Geometry: final body of the model. Coordinates: model frame, mm. Round coordinates to 2 decimals unless told otherwise and drop trailing zeros. Write each loop counter-clockwise with the first axis right and the second up, starting at its lowest first coordinate (ties: lowest second). Pieces come first, ordered by that corner, then holes. Notation, with made-up numbers: M -36.5,47 L 2.5,47 A20 ccw 2.5,75 Z; hole C -18.5,-34.5 d9. An arc over 180 degrees is marked long. Use one line per item in the form item = value. Start each with the question number.
Autodesk Inventor part; units mm, degrees
ref_plane "YZ Plane" through (0, 0, 0) normal (1, 0, 0) x (0, 1, 0)
ref_plane "XZ Plane" through (0, 0, 0) normal (0, 1, 0) x (-1, 0, 0)
ref_plane "XY Plane" through (0, 0, 0) normal (0, 0, 1) x (1, 0, 0)
sketch "Sketch1" plane through (0, 0, 0) normal (0, 0, 1) x (1, 0, 0)
  line L0 (0, 22.2362) -> (22.2362, 22.2362) construction
  line L1 (22.2362, 22.2362) -> (22.2362, 0) construction
  line L2 (22.2362, 0) -> (0, 0)
  line L3 (0, 0) -> (0, 22.2362)
  line L4 (0, 22.2362) -> (22.2362, 0) construction
  line L5 (22.2362, 22.2362) -> (0, 0) construction
  line L6 (208.1103, 421.1181) -> (230.3465, 421.1181)
  line L7 (230.3465, 421.1181) -> (230.3465, 398.8819)
  line L8 (230.3465, 398.8819) -> (208.1103, 398.8819) construction
  line L9 (208.1103, 398.8819) -> (208.1103, 421.1181) construction
  line L10 (208.1103, 421.1181) -> (230.3465, 398.8819) construction
  line L11 (230.3465, 421.1181) -> (208.1103, 398.8819) construction
  line L12 (208.1103, 421.1181) -> (0, 22.2362)
  line L13 (230.3465, 398.8819) -> (22.2362, 0)
  line L14 (0, 0) -> (230.3465, 421.1181) construction
  line L15 (-46.0693, 0) -> (276.4159, 0) construction
  point P0 (11.1181, 11.1181)
  point P1 (219.2284, 410)
  point P2 (115.1733, 210.5591)
  dimension "d1" = 480
  dimension "d14" = 410
  dimension "d15" = 30
extrude "Extrusion1" add sketch "Sketch1" along normal mid plane 10
sketch "Sketch2" plane through (0, 0, 5) normal (0, 0, 1) x (1, 0, 0)
  line L0 (230.3465, 421.1181) -> (208.1103, 421.1181) construction
  line L1 (230.3465, 398.8819) -> (230.3465, 421.1181) construction
  line L2 (208.1103, 421.1181) -> (230.3465, 398.8819) construction
  point P0 (0, 0)
  point P1 (219.2284, 410)
hole "Hole1" at (219.2284, 410, 5) direction (0, 0, -1) diameter 8 end through all
properties part number "Support - Left"
1. Section query D-D (y = 269). Return loops of the section in (x, z), then the cut area to 3 significant figures.
2. Section query C-C (x = 195). Return loops of the section in (y, z), then the cut area to 3 significant figures.
3. Ray query, probe 1 along X at (y, z) = (410, 1); probe 2 along X at (y, z) = (207, 2.25); probe 3 along Y at (x, z) = (67, 3.25). Return the intervals inside material, ascending.
4. Pull-direction query (Y, two-part tool) for faces 1 (the face through (11, 0, 0)), 2 (the face through (115, 212, 5)), 3 (the face through (219.053, 413.996, -0.07)), 4 (the face through (219, 421.118, 0)); classes: released by +Y, released by -Y, zero draft, split by the parting line, or undercut.
5. Section query A-A (y = 410). Return loops of the section in (x, z), then the cut area to 3 significant figures.
6. Section query B-B (z = 1.25). Return loops of the section in (x, y), then the cut area to 3 significant figures.
7. Contact query for flat-ended pins moving along their axis: pin 1 (1.5 mm diameter, centred on x = 142, z = -1.5, fed in from -Y); pin 2 (4 mm diameter, centred on x = 187.5, z = 0, fed in from -Y); pin 3 (2 mm diameter, centred on y = 258, z = -1.5, fed in from +X); pin 4 (10.5 mm diameter, centred on x = 219.23, y = 410, fed in from -Z). Output: stop coordinate, or through.
Checks:
q1.outline = M 128.75,-5 L 162.58,-5 L 162.58,5 L 128.75,5 Z
q1.area = 338 mm^2
q2.outline = M 331.13,-5 L 395.99,-5 L 395.99,5 L 331.13,5 Z
q2.area = 649 mm^2
q3.probe_1 = 202.31 to 215.23, 223.23 to 230.35
q3.probe_2 = 96.4 to 130.24
q3.probe_3 = 85.8 to 150.65
q4.face_1 = released by -Y
q4.face_2 = zero draft
q4.face_3 = undercut
q4.face_4 = released by +Y
q5.outline = M 202.31,-5 L 215.23,-5 L 215.23,5 L 202.31,5 Z; M 223.23,-5 L 230.35,-5 L 230.35,5 L 223.23,5 Z
q5.area = 200 mm^2
q6.outline = M 0,0 L 22.24,0 L 230.35,398.88 L 230.35,421.12 L 208.11,421.12 L 0,22.24 Z; hole C 219.23,410 d8
q6.area = 13,900 mm^2
q7.pin_1 = 228.11
q7.pin_2 = 312.93
q7.pin_3 = 157.37
q7.pin_4 = -5
